```python
from build123d import *

# Parameters (mm, degrees)
F0_W     = 9.6774
F0_H     = 33.528
F0_W_2   = 6.7188069224
F0_H_2   = 4.5997034758
F0_W_3   = 23.2836488279
F0_W_4   = 5.7477712986
F0_H_3   = 13.2390651852
F1_DEPTH = 3.5


with BuildPart() as f1:
    # F0 (on Top) → F1 (new body)
    with BuildSketch(Plane.XY):
        with Locations((-34.2135546392, 25.1117386506)):
            Rectangle(F0_W, F0_H)
        with BuildLine():
            ThreePointArc((-29.3748546392, 41.8757386506), (-0.8171033114, 68.9673107238), (27.7406480163, 41.8757386506))
            Line((27.7406480163, 41.8757386506), (37.4212376773, 41.8757386506))
            ThreePointArc((37.4212376773, 41.8757386506), (-0.8155084809, 76.4992777712), (-39.0522546392, 41.8757386506))
            Line((-39.0522546392, 41.8757386506), (-29.3748546392, 41.8757386506))
        make_face()
        Polygon((27.7406480163, 41.8757386506), (27.7406480163, 8.341178298), (37.4212376773, 8.3477386506), (37.4212376773, 41.8757386506), align=None)
        with BuildLine():
            ThreePointArc((27.7406480163, 8.341178298), (27.6786104385, 6.4663822858), (27.4936267406, 4.5997034758))
            ThreePointArc((27.4936267406, 4.5997034758), (27.0884181011, 2.2792068562), (26.4933427197, 0))
            ThreePointArc((26.4933427197, 0), (-0.8171029347, -20.210013054), (-28.127548589, 0))
            ThreePointArc((-28.127548589, 0), (-28.7226239704, 2.2792068562), (-29.1278326099, 4.5997034758))
            ThreePointArc((-29.1278326099, 4.5997034758), (-29.3130322146, 6.4696553488), (-29.3748546392, 8.3477386506))
            Line((-29.3748546392, 8.3477386506), (-39.0522546392, 8.3477386506))
            ThreePointArc((-39.0522546392, 8.3477386506), (-0.8155084809, -29.8890075077), (37.4212376773, 8.3477386506))
            Line((37.4212376773, 8.3477386506), (27.7406480163, 8.341178298))
        make_face()
        with BuildLine():
            Line((27.4936267406, 4.5997034758), (16.9359110296, 4.5997034758))
            Line((16.9359110296, 4.5997034758), (16.9359110296, 0))
            Line((16.9359110296, 0), (26.4933427197, 0))
            ThreePointArc((26.4933427197, 0), (27.0884181011, 2.2792068562), (27.4936267406, 4.5997034758))
        make_face()
        with Locations((13.5765075684, 2.2998517379)):
            Rectangle(F0_W_2, F0_H_2)
        with Locations((-1.4247203068, 2.2998517379)):
            Rectangle(F0_W_3, F0_H_2)
        with Locations((-15.9404303701, 2.2998517379)):
            Rectangle(F0_W_4, F0_H_2)
        with BuildLine():
            Line((-18.8143160194, 0), (-18.8143160194, 4.5997034758))
            Line((-18.8143160194, 4.5997034758), (-29.1278326099, 4.5997034758))
            ThreePointArc((-29.1278326099, 4.5997034758), (-28.7226239704, 2.2792068562), (-28.127548589, 0))
            Line((-28.127548589, 0), (-18.8143160194, 0))
        make_face()
        with BuildLine():
            ThreePointArc((-13.0665447208, 41.155968661), (-1.5272068761, 54.4534372667), (10.792715475, 41.8757386506))
            Line((10.792715475, 41.8757386506), (10.2171041071, 17.838768661))
            Line((10.2171041071, 17.838768661), (16.9359110296, 17.838768661))
            Line((16.9359110296, 17.838768661), (16.2751674652, 41.8757386506))
            ThreePointArc((16.2751674652, 41.8757386506), (-1.1801254004, 59.0346097607), (-18.6354182661, 41.8757386506))
            Line((-18.6354182661, 41.8757386506), (-18.8143160194, 17.838768661))
            Line((-18.8143160194, 17.838768661), (-13.0665447208, 17.838768661))
            Line((-13.0665447208, 17.838768661), (-13.0665447208, 41.155968661))
        make_face()
        with Locations((13.5765075684, 11.2192360684)):
            Rectangle(F0_W_2, F0_H_3)
        with Locations((-15.9404303701, 11.2192360684)):
            Rectangle(F0_W_4, F0_H_3)
        with BuildLine():
            Line((10.2171041071, 17.838768661), (10.792715475, 41.8757386506))
            ThreePointArc((10.792715475, 41.8757386506), (-1.5272068761, 54.4534372667), (-13.0665447208, 41.155968661))
            Line((-13.0665447208, 41.155968661), (-13.0665447208, 17.838768661))
            Line((-13.0665447208, 17.838768661), (-13.0665447208, 4.5997034758))
            Line((-13.0665447208, 4.5997034758), (10.2171041071, 4.5997034758))
            Line((10.2171041071, 4.5997034758), (10.2171041071, 17.838768661))
        make_face()
        with BuildLine():
            Line((16.9359110296, 0), (10.2171041071, 0))
            Line((10.2171041071, 0), (-13.0665447208, 0))
            Line((-13.0665447208, 0), (-18.8143160194, 0))
            Line((-18.8143160194, 0), (-28.127548589, 0))
            ThreePointArc((-28.127548589, 0), (-0.8171029347, -20.210013054), (26.4933427197, 0))
            Line((26.4933427197, 0), (16.9359110296, 0))
        make_face()
    extrude(amount=F1_DEPTH)


solid = f1.part
```
The listing builds one solid part. Answer for the finished solid, in the listing's coordinates (mm). A direction names the side the tool comes from. Round coordinates to 2 decimals unless told otherwise and drop trailing zeros. Loops run counter-clockwise (first coordinate to the right, second up) from the corner with the lowest first, then second, coordinate; pieces in that order, holes last.
Q1. Given pin 1 Ø1 at (x, y) = (-20, 6) entering from +Z, flat-ended and moving along its own axis, determine where the tip first touches the part or whether it passes through.
Q2. Section D-D, the plane y = 47 is taken. Determine the outline of the cut face in (x, z), then the cut area to 3 significant figures.
Q3. Find the intervals of material crossed by line 1 (X direction, y = 34.5, z = 2.15); line 2 (X direction, y = 22.5, z = 1.35); line 3 (Y direction, x = 10.5, z = 1.2), in increasing order.
Q4. Which of the six approach directions +Z, -Z, +X, -X, +Y, -Y give full straight-line access (tool end or side, diameter ignored) to faces 5 (the face through (-29.31, 6.44, 1.73)), 6 (the face through (-1.66, -29.88, 1.73))?
Q5. Section C-C, the plane x = 19 is taken. Determine the outline of the cut face in (y, z).
Q6. For a pull along X with two mould halves and no side action, classify faces 1 (the face through (-1.42, 68.96, 1.73)), 2 (the face through (-1, 24, 0)), 3 (the face through (-39.052, 25, 2)), 4 (the face through (27.741, 25, 2)) as released by +X, released by -X, zero draft, split by the parting line, or undercut.
Q7. Section A-A, the plane y = 10.5 is taken. Determine the outline of the cut face in (x, z).
Completed:
1. pin 1: passes through
2. outline: (-38.19, 0) - (-28.64, 0) - (-28.64, 3.5) - (-38.19, 3.5) - close; (-17.77, 0) - (15.41, 0) - (15.41, 3.5) - (-17.77, 3.5) - close; (27, 0) - (36.56, 0) - (36.56, 3.5) - (27, 3.5) - close
2. area: 183 mm2
3. line 1: x = -39.05 to -29.37, -18.69 to 16.48, 27.74 to 37.42
3. line 2: x = -39.05 to -29.37, -18.78 to 16.81, 27.74 to 37.42
3. line 3: y = -28.18 to 54.55, 66.63 to 74.8
4. face 5: +Z, -Z
4. face 6: +Z, -Z, -Y
5. outline: (-24.35, 0) - (4.6, 0) - (4.6, 3.5) - (-24.35, 3.5) - close; (60.99, 0) - (71, 0) - (71, 3.5) - (60.99, 3.5) - close
6. face 1: undercut
6. face 2: zero draft
6. face 3: released by -X
6. face 4: undercut
7. outline: (-39.05, 0) - (-29.37, 0) - (-29.37, 3.5) - (-39.05, 3.5) - close; (-18.81, 0) - (16.94, 0) - (16.94, 3.5) - (-18.81, 3.5) - close; (27.74, 0) - (37.42, 0) - (37.42, 3.5) - (27.74, 3.5) - close
